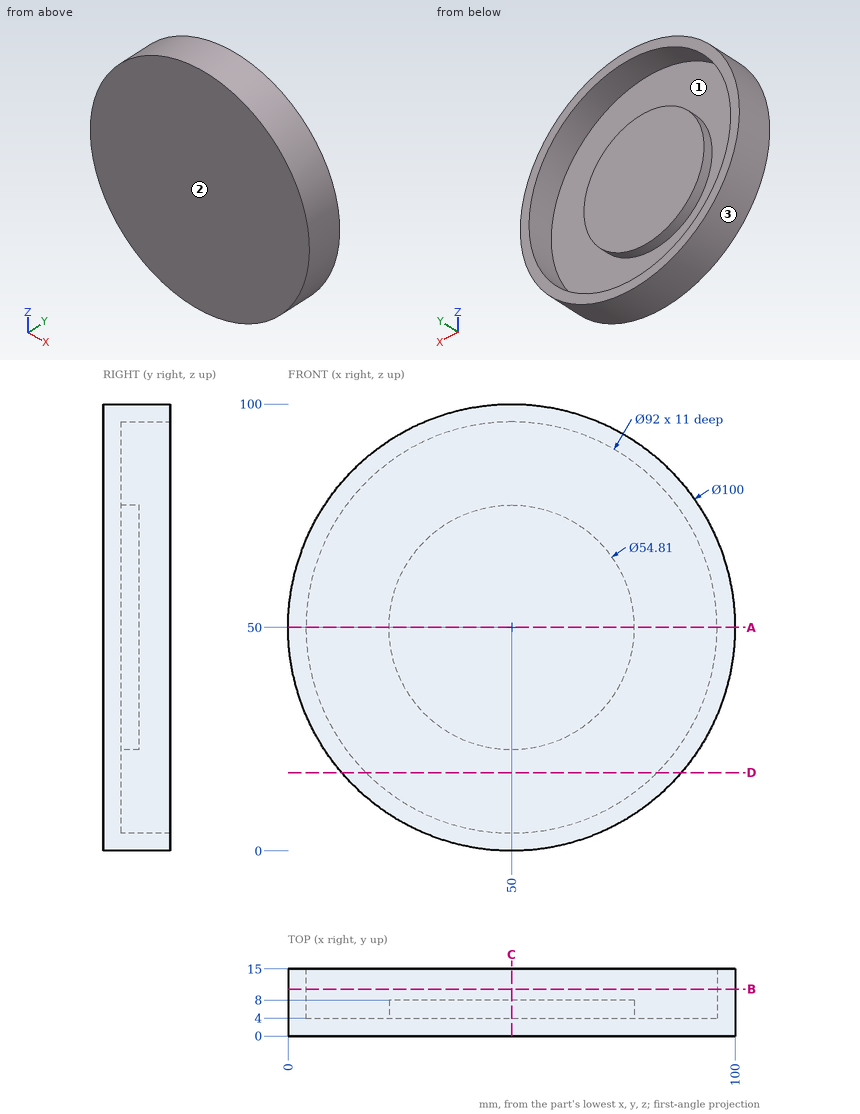
Print and shaded views of the part. All mm, measured from the part's lowest x, y and z. Give positions to 0.01 mm unless a question says otherwise; leave off trailing zeros. Loops run counter-clockwise (first coordinate to the right, second up) from the corner with the lowest first, then second, coordinate; pieces in that order, holes last.
1) Wall check: line 1 (X direction, y = 7.75, z = 50) (3 decimals); line 2 (X direction, y = 11, z = 50); line 3 (X direction, y = 7.75, z = 34.5). Give the ranges that are in metal, low to high.
2) Flat gauge pins, fed straight in: pin 1 Ø12 at (x, z) = (45, 45) entering from +Y; pin 2 Ø4 at (x, y) = (80.5, 4.5) entering from -Z; pin 3 Ø8 at (x, z) = (41.5, 70.5) entering from -Y; pin 4 Ø8 at (x, z) = (18.5, 73.5) entering from +Y. Where does each tip first touch, or does it go through?
3) Saw through at B-B (y = 10.5). Write the cut outline in (x, z).
4) Saw through at C-C (x = 50). Write the cut outline in (y, z) (3 decimals), plus the area to 3 significant figures.
5) Saw through at D-D (z = 17.5). Write the cut outline in (x, y), plus the area to 3 significant figures.
6) Pull direction Z, two halves, no side cores. Call the marked faces 1, 2 and 3: +Z half, -Z half, draft (parallel to the pull), parting line (faces both ways), or undercut.
7) Saw through at A-A (z = 50). Write the cut outline in (x, y) (3 decimals), plus the area to 3 significant figures.
Answer block:
1. line 1: x = 0 to 4, 22.595 to 77.405, 96 to 100
1. line 2: x = 0 to 4, 96 to 100
1. line 3: x = 2.46 to 6.69, 27.4 to 72.6, 93.31 to 97.54
2. pin 1: stops at y = 8
2. pin 2: stops at z = 8.92
2. pin 3: stops at y = 0
2. pin 4: stops at y = 4
3. outline: circle Ø100 at (50, 50); hole circle Ø92 at (50, 50)
4. outline: (0, 0) - (15, 0) - (15, 4) - (4, 4) - (4, 22.595) - (8, 22.595) - (8, 77.405) - (4, 77.405) - (4, 96) - (15, 96) - (15, 100) - (0, 100) - close
4. area: 707 mm2
5. outline: (12, 0) - (88, 0) - (88, 15) - (82.55, 15) - (82.55, 4) - (17.45, 4) - (17.45, 15) - (12, 15) - close
5. area: 424 mm2
6. face 1: undercut
6. face 2: draft
6. face 3: parting line
7. outline: (0, 0) - (100, 0) - (100, 15) - (96, 15) - (96, 4) - (77.405, 4) - (77.405, 8) - (22.595, 8) - (22.595, 4) - (4, 4) - (4, 15) - (0, 15) - close
7. area: 707 mm2
